The model under review builds one solid part; all positions refer to its coordinate system, in mm. A direction names the side the tool comes from. Round coordinates to 2 decimals unless told otherwise and drop trailing zeros. Order: outer loops, then holes, each group sorted by start corner. A loop starts at its lowest first (then second) coordinate and runs counter-clockwise, first axis right, second up.
1) Machinability: for faces 4 (the face through (42, 17, 2)), 5 (the face through (0, -3, 2)), which of the approach directions +Z, -Z, +X, -X, +Y, -Y give a long, thin tool a straight path to every point of the face, cutting with its end or side? Answer none if there is none.
2) To check wall thickness, follow L1, parallel to Y at x = 42, z = 3.9; L2, parallel to X at y = -1.5, z = 3.15; L3, parallel to Y at x = 6.5, z = 4.55 (3 decimals). State the ranges of each line that lie inside material, in increasing order.
3) Mouldability with a two-part tool opening along Y and no side actions: class faces 1 (the face through (27, 10, 5)), 2 (the face through (30, 0, 2)), 3 (the face through (42, 34, 2)) as pulls with the +Y half, pulls with the -Y half, needs draft (parallel to the pull), parting line crosses it, or undercut.
4) Consider section A-A (z = 0.7). Give the boundary of the cut face in (x, y), then the cut area to 3 significant figures.
5) Clearance check with flat-ended pins moving along their axes: P1, Ø1.5, axis at y = -3.5, z = 3.5, coming from the +X side; P2, Ø1.5, axis at x = 43.5, z = 2, coming from the -Y side; P3, Ø1.5, axis at x = 26.5, z = 3.5, coming from the -Y side. State where each tip first meets the part, or that it passes through.
6) Consider section C-C (y = -2). Give the boundary of the cut face in (x, z).
7) Consider section B-B (x = 41.5). Give the boundary of the cut face in (y, z), then the cut area to 3 significant figures.
from build123d import *

# Parameters (mm, degrees)
CROQUIS1_W              = 5
CROQUIS1_H              = 17
CROQUIS1_W_2            = 20
CROQUIS1_H_2            = 5
SALIENTE_EXTRUIR1_DEPTH = 5


with BuildPart() as part:
    # Croquis1 → Saliente-Extruir1 (new body)
    with BuildSketch(Plane.XY):
        with Locations((42.5, 25.5)):
            Rectangle(CROQUIS1_W, CROQUIS1_H)
        Polygon((40, 0), (0, 0), (40, 34), align=None)
        with Locations((10, -2.5)):
            Rectangle(CROQUIS1_W_2, CROQUIS1_H_2)
    extrude(amount=SALIENTE_EXTRUIR1_DEPTH)


solid = part.part
Answer below:
1. face 4: +Z, -Z, +X, -Y
1. face 5: +Z, -Z, -X, +Y, -Y
2. L1: y = 17 to 34
2. L2: x = 0 to 20
2. L3: y = -5 to 5.525
3. face 1: needs draft
3. face 2: pulls with the -Y half
3. face 3: pulls with the +Y half
4. outline: (0, -5) - (20, -5) - (20, 0) - (40, 0) - (40, 17) - (45, 17) - (45, 34) - (40, 34) - (0, 0) - close
4. area: 865 mm2
5. P1: stops at x = 20
5. P2: stops at y = 17
5. P3: stops at y = 0
6. outline: (0, 0) - (20, 0) - (20, 5) - (0, 5) - close
7. outline: (17, 0) - (34, 0) - (34, 5) - (17, 5) - close
7. area: 85.0 mm2
